Geometry check sheet. Reference: the model listing, model coordinates, mm. Give positions to 0.01 mm unless a question says otherwise; leave off trailing zeros. Loops run counter-clockwise (first coordinate to the right, second up) from the corner with the lowest first, then second, coordinate; pieces in that order, holes last. Notation, with made-up numbers: (-36, 88) -> (1, 88) arc R18 ccw to (1, 102) -> close; hole circle Ø9 at (24.25, -21.75). An arc over 180 degrees is marked (long way). Write each question's results on one line, items separated by ' | '. Start each with the question number.
1) Scan lines: line 1 (X direction, y = 8.3, z = -100); line 2 (X direction, y = 7.5, z = -95.5); line 3 (Z direction, x = 172, y = 6.5). Record each from-to range of solid material in increasing order. Write a range as from..to.
2) Sectioned sample at B-B on z = -94. Record the cut outline in (x, y), then the cut area to 3 significant figures.
3) Depth check by flat-ended pin: pin 1 (4 mm diameter, centred on x = 123.5, z = -165.5, fed in from -Y). Enter the tip coordinate at first touch or a pass-through.
4) Sectioned sample at C-C on x = 183. Record the cut outline in (y, z).
5) Sectioned sample at A-A on y = 7.75. Record the cut outline in (x, z), then the cut area to 3 significant figures.
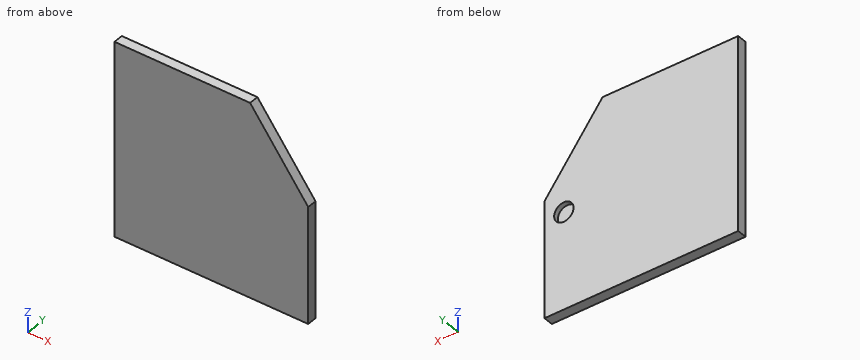
```python
from build123d import *

# Parameters (mm, degrees)
EXTRUDE_1_DEPTH     = 10
SKETCH_2_R          = 10
CUT_EXTRUDE_1_DEPTH = 5


with BuildPart() as part:
    # Эскиз1 → Бобышка-Вытянуть1 (new body)
    with BuildSketch(Plane(origin=(0, 0, 0), x_dir=(1, 0, 0), z_dir=(0, 1, 0))):
        Polygon((0, 0), (140, 0), (200, 80), (200, 120), (200, 200), (140, 200), (0, 200), align=None)
    extrude(amount=EXTRUDE_1_DEPTH)

    # Эскиз2 → Вырез-Вытянуть1 (cut)
    with BuildSketch(Plane(origin=(0, 10, 0), x_dir=(1, 0, 0), z_dir=(0, 1, 0))):
        with Locations(Location((180, 100, 0), (0, 0, 270))):
            Circle(SKETCH_2_R)
    extrude(amount=-CUT_EXTRUDE_1_DEPTH, mode=Mode.SUBTRACT)


solid = part.part
```
Result:
1) line 1: 0..170, 190..200 | line 2: 0..171.07, 188.93..200 | line 3: -200..-106, -94..-42.67
2) outline: (0, 0) -> (200, 0) -> (200, 10) -> (188, 10) -> (188, 5) -> (172, 5) -> (172, 10) -> (0, 10) -> close | area: 1,920 mm^2
3) pin 1: y = 0
4) outline: (0, -200) -> (10, -200) -> (10, -109.54) -> (5, -109.54) -> (5, -90.46) -> (10, -90.46) -> (10, -57.33) -> (0, -57.33) -> close
5) outline: (0, -200) -> (200, -200) -> (200, -80) -> (140, 0) -> (0, 0) -> close; hole circle Ø20 at (180, -100) | area: 37,300 mm^2
